Build history of the part. All positions in model axes, mm. A direction names the side the tool comes from. Give positions to 0.01 mm unless a question says otherwise; leave off trailing zeros. Write each loop counter-clockwise with the first axis right and the second up, starting at its lowest first coordinate (ties: lowest second). Pieces come first, ordered by that corner, then holes. Notation, with made-up numbers: M 34.25,13.25 L 91.25,13.25 A11 cw 91.25,20.25 Z; hole C -25,70.25 d1. An arc over 180 degrees is marked long. Return JSON: item names as keys, results as strings. Group by question number.
Q1. Flat gauge pins, fed straight in: pin 1 Ø2 at (x, y) = (10, 10) entering from +Z; pin 2 Ø1.5 at (x, y) = (-17.5, -13.5) entering from -Z; pin 3 Ø6 at (x, z) = (-2.5, -9.5) entering from +Y. Where does each tip first touch, or does it go through?
Q2. Wall check: probe 1 along X at (y, z) = (10, 1.55); probe 2 along Y at (x, z) = (0, -5.25). Give the ranges that are in metal, low to high.
Q3. Band-saw the part on A-A, the plane y = 0. Give the cut face in (x, z).
Q4. Pull direction Y, two halves, no side cores. Call faces 3 (the cylindrical face through (1.08, -4.88, -7.6)), 4 (the flat face through (-25, 0, 2)), 5 (the flat face through (0, -25, 2)): +Y half, -Y half, draft (parallel to the pull), parting line (faces both ways), or undercut.
Q5. Band-saw the part on D-D, the plane y = 11. Give the cut face in (x, z), then the cut area to 3 significant figures.
Q6. Tool access for faces 1 (the flat face through (25, 0, 2)), 2 (the flat face through (-17, 11, 0)): list every direction of +Z, -Z, +X, -X, +Y, -Y with a clear straight run to the whole face (end or side of a thin tool).
from build123d import *
from build123d.topology import SkipClean

# Parameters (mm, degrees)
SKETCH_1_W      = 50
SKETCH_1_H      = 50
SKETCH_1_R      = 1.65
EXTRUDE_1_DEPTH = 5
EXTRUDE_START   = 15
SKETCH_4_R      = 18.5
SKETCH_4_R_2    = 1.65
SKETCH_4_R_3    = 5
EXTRUDE_4_DEPTH = 15


with BuildPart() as part:
    # 草图1 → 凸台-拉伸1 (new body)
    with BuildSketch(Plane.XY):
        Rectangle(SKETCH_1_W, SKETCH_1_H)
        with Locations((-10, 10)):
            Circle(SKETCH_1_R, mode=Mode.SUBTRACT)
        with Locations((0, 10)):
            Circle(SKETCH_1_R, mode=Mode.SUBTRACT)
        with Locations((-10, 0)):
            Circle(SKETCH_1_R, mode=Mode.SUBTRACT)
        with Locations(Location((-10, -10, 0), (0, 0, 180))):
            Circle(SKETCH_1_R, mode=Mode.SUBTRACT)
        with Locations(Location((0, -10, 0), (0, 0, 180))):
            Circle(SKETCH_1_R, mode=Mode.SUBTRACT)
        with Locations((10, -10)):
            Circle(SKETCH_1_R, mode=Mode.SUBTRACT)
        with Locations(Location((10, 0, 0), (0, 0, 180))):
            Circle(SKETCH_1_R, mode=Mode.SUBTRACT)
        with Locations(Location((10, 10, 0), (0, 0, 180))):
            Circle(SKETCH_1_R, mode=Mode.SUBTRACT)
    extrude(amount=EXTRUDE_1_DEPTH)

    # 草图4 → 凸台-拉伸4 (add)
    with SkipClean():  # the faces are left unmerged after this step: merging them gives an invalid solid
        with BuildSketch(Plane(origin=(0, 0, 0), x_dir=(-1, 0, 0), z_dir=(0, 0, -1)).offset(EXTRUDE_START)):
            Circle(SKETCH_4_R)
            with Locations((10, -10)):
                Circle(SKETCH_4_R_2, mode=Mode.SUBTRACT)
            with Locations((0, -10)):
                Circle(SKETCH_4_R_2, mode=Mode.SUBTRACT)
            with Locations((-10, -10)):
                Circle(SKETCH_4_R_2, mode=Mode.SUBTRACT)
            with Locations((10, 0)):
                Circle(SKETCH_4_R_2, mode=Mode.SUBTRACT)
            with Locations((-10, 0)):
                Circle(SKETCH_4_R_2, mode=Mode.SUBTRACT)
            with Locations((10, 10)):
                Circle(SKETCH_4_R_2, mode=Mode.SUBTRACT)
            with Locations((0, 10)):
                Circle(SKETCH_4_R_2, mode=Mode.SUBTRACT)
            Circle(SKETCH_4_R_3, mode=Mode.SUBTRACT)
            with Locations((-10, 10)):
                Circle(SKETCH_4_R_2, mode=Mode.SUBTRACT)
        extrude(amount=-EXTRUDE_4_DEPTH)


solid = part.part
From the geometry:
{
 "1": {"pin 1": "passes through", "pin 2": "stops at z = 0", "pin 3": "stops at y = 18.5"},
 "2": {"probe 1": "x = -25 to -11.65, -8.35 to -1.65, 1.65 to 8.35, 11.65 to 25", "probe 2": "y = -18.5 to -11.65, -8.35 to -5, 5 to 8.35, 11.65 to 18.5"},
 "3": {"outline": "M -25,0 L -18.5,0 L -18.5,-15 L -11.65,-15 L -11.65,5 L -25,5 Z; M -8.35,-15 L -5,-15 L -5,0 L 5,0 L 5,-15 L 8.35,-15 L 8.35,5 L -8.35,5 Z; M 11.65,-15 L 18.5,-15 L 18.5,0 L 25,0 L 25,5 L 11.65,5 Z"},
 "4": {"face 3": "undercut", "face 4": "draft", "face 5": "-Y half"},
 "5": {"outline": "M -25,0 L -14.87,0 L -14.87,-15 L -11.31,-15 L -11.31,5 L -25,5 Z; M -8.69,-15 L -1.31,-15 L -1.31,5 L -8.69,5 Z; M 1.31,-15 L 8.69,-15 L 8.69,5 L 1.31,5 Z; M 11.31,-15 L 14.87,-15 L 14.87,0 L 25,0 L 25,5 L 11.31,5 Z", "area": "539 mm^2"},
 "6": {"face 1": "+Z, -Z, +X, +Y, -Y", "face 2": "-Z"}
}
